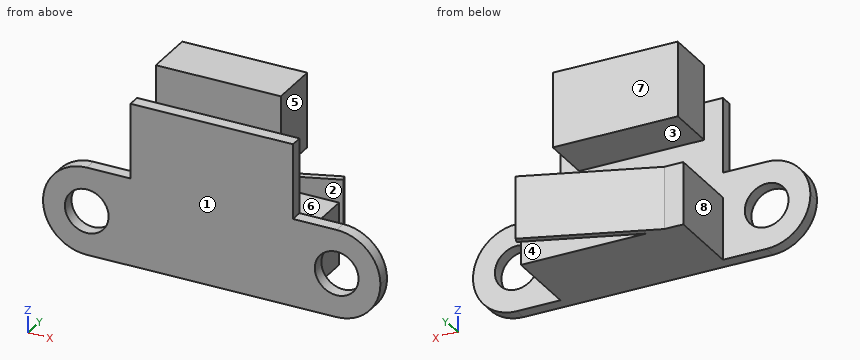
from build123d import *

# Parameters (mm, degrees)
SKETCH1_W           = 13
SKETCH1_H           = 13
BOSS_EXTRUDE1_DEPTH = 1
SKETCH4_W           = 7
SKETCH4_H           = 1
BOSS_EXTRUDE2_DEPTH = 7
SKETCH5_W           = 7
SKETCH5_H           = 1
BOSS_EXTRUDE3_DEPTH = 7
SKETCH6_R           = 1.75
CUT_EXTRUDE1_DEPTH  = 16.016657418
SKETCH7_W           = 10
SKETCH7_H           = 6
BOSS_EXTRUDE4_DEPTH = 4
SKETCH8_W           = 13
SKETCH8_H           = 5
BOSS_EXTRUDE5_DEPTH = 6
BOSS_EXTRUDE6_DEPTH = 5
FILLET1_R           = 3.5


with BuildPart() as part:
    # Sketch1 → Boss-Extrude1 (new body)
    with BuildSketch(Plane(origin=(0, 0, 0), x_dir=(1, 0, 0), z_dir=(0, 1, 0))):
        Rectangle(SKETCH1_W, SKETCH1_H)
    extrude(amount=BOSS_EXTRUDE1_DEPTH)

    # Sketch4 → Boss-Extrude2 (add)
    with BuildSketch(Plane.ZY.offset(6.5)):
        with Locations((-3, 0.5)):
            Rectangle(SKETCH4_W, SKETCH4_H)
    extrude(amount=BOSS_EXTRUDE2_DEPTH)

    # Sketch5 → Boss-Extrude3 (add)
    with BuildSketch(Plane(origin=(6.5, 0, 0), x_dir=(0, 0, -1), z_dir=(1, 0, 0))):
        with Locations((3, 0.5)):
            Rectangle(SKETCH5_W, SKETCH5_H)
    extrude(amount=BOSS_EXTRUDE3_DEPTH)

    # Sketch6 → Cut-Extrude1 (cut, through all)
    with BuildSketch(Plane(origin=(0, 1, 0), x_dir=(1, 0, 0), z_dir=(0, 1, 0))):
        with Locations(Location((-10, 3, 0), (0, 0, 270))):
            Circle(SKETCH6_R)
        with Locations(Location((10, 3, 0), (0, 0, 270))):
            Circle(SKETCH6_R)
    extrude(amount=-CUT_EXTRUDE1_DEPTH, mode=Mode.SUBTRACT)

    # Sketch7 → Boss-Extrude4 (add)
    with BuildSketch(Plane(origin=(0, 1, 0), x_dir=(1, 0, 0), z_dir=(0, 1, 0))):
        with Locations((0, -6.5)):
            Rectangle(SKETCH7_W, SKETCH7_H)
    extrude(amount=BOSS_EXTRUDE4_DEPTH)

    # Sketch8 → Boss-Extrude5 (add)
    with BuildSketch(Plane(origin=(0, 1, 0), x_dir=(1, 0, 0), z_dir=(0, 1, 0))):
        with Locations((0, 4)):
            Rectangle(SKETCH8_W, SKETCH8_H)
    extrude(amount=BOSS_EXTRUDE5_DEPTH)

    # Sketch9 → Boss-Extrude6 (add)
    with BuildSketch(Plane.XY.offset(-1.5)):
        Polygon((-5, 7), (5, 10.639702343), (5.171010072, 10.169856032), (-3.5380978, 7), align=None)
    extrude(amount=-BOSS_EXTRUDE6_DEPTH)

    # Fillet1
    fillet1_edges = [part.edges().sort_by_distance(p)[0] for p in [
        (13.5, 0.5, -6.5),
        (13.5, 0.5, 0.5),
        (-13.5, 0.5, -6.5),
        (-13.5, 0.5, 0.5),
    ]]
    fillet(fillet1_edges, radius=FILLET1_R - 0.0001)  # a hair under: the kernel refuses the full size


solid = part.part
Can you work these out from the model? Positions are in its coordinate system, mm. Face numbers are marked on the shaded views. A direction names the side the tool comes from. Give positions to 0.01 mm unless a question says otherwise; leave off trailing zeros. Order: outer loops, then holes, each group sorted by start corner. A loop starts at its lowest first (then second) coordinate and runs counter-clockwise, first axis right, second up. Notation, with made-up numbers: (86, 6.25) - (108, 6.25) arc R21 ccw to (108, 24.25) - close; hole circle Ø8 at (14, 15.5). An arc over 180 degrees is marked (long way). Write each question's results on one line, items separated by ' | '.
1) If we mould it in two halves opening along Y, with no side actions, what happens to the marked faces 1, 2, 3 and 4? For each: pulls with the +Y half, pulls with the -Y half, needs draft (parallel to the pull), parting line crosses it, or undercut.
Final values:
face 1: pulls with the -Y half | face 2: undercut | face 3: needs draft | face 4: undercut
2) I'm going to push flat-ended pins straight in: pin 1 Ø3 at (x, y) = (6, 1) entering from +Z; pin 2 Ø1.8 at (x, z) = (0, 6) entering from +Y; pin 3 Ø1.5 at (x, z) = (1, 7.5) entering from -Y; pin 4 Ø4 at (y, z) = (7, 3) entering from -X. Where does each tip first touch, or does it pass through?
Final values:
pin 1: stops at z = 9.5 | pin 2: stops at y = 5 | pin 3: stops at y = 1 | pin 4: passes through
3) Suppose I cut it at B-B, the plane z = -4. Write out the boundary of the cut face in (x, y).
Final values:
outline: (-13.35, 0) - (-11.44, 0) - (-11.44, 1) - (-13.35, 1) - close; (-8.56, 0) - (8.56, 0) - (8.56, 1) - (6.5, 1) - (6.5, 7) - (-3.54, 7) - (5.17, 10.17) - (5, 10.64) - (-5, 7) - (-6.5, 7) - (-6.5, 1) - (-8.56, 1) - close; (11.44, 0) - (13.35, 0) - (13.35, 1) - (11.44, 1) - close
4) Suppose I cut it at C-C, the plane y = 5.75. Write out the boundary of the cut face in (x, z), then the cut area to 3 significant figures.
Final values:
outline: (-6.5, -6.5) - (6.5, -6.5) - (6.5, -1.5) - (-6.5, -1.5) - close | area: 65.0 mm^2
5) Suppose I cut it at D-D, the plane x = 10.5. Write out the boundary of the cut face in (y, z).
Final values:
outline: (0, -6.46) - (1, -6.46) - (1, -4.68) - (0, -4.68) - close; (0, -1.32) - (1, -1.32) - (1, 0.46) - (0, 0.46) - close
6) Please list where these lines run through material, in increasing order: line 1 along X through (y, z) = (0.75, -3); line 2 along X through (y, z) = (3, 8); line 3 along Y through (x, z) = (4.5, 2.75). Write a range as [from, to].
Final values:
line 1: x = [-13.5, -11.75], [-8.25, 8.25], [11.75, 13.5] | line 2: x = [-5, 5] | line 3: y = [0, 1]
7) Suppose I cut it at A-A, the plane x = 4.25. Write out the boundary of the cut face in (y, z), then the cut area to 3 significant figures.
Final values:
outline: (0, -6.5) - (7, -6.5) - (7, -1.5) - (1, -1.5) - (1, 3.5) - (5, 3.5) - (5, 9.5) - (1, 9.5) - (1, 6.5) - (0, 6.5) - close; (9.83, -6.5) - (10.37, -6.5) - (10.37, -1.5) - (9.83, -1.5) - close | area: 69.7 mm^2
8) On a 3-axis mill with a long thin cutter (end or side, diameter ignored), from which of +Z, -Z, +X, -X, +Y, -Y can I reach the whole of each face in a straight line? I mean the marked faces 5, 6, 7 and 8. Say none if no direction works.
Final values:
face 5: +Z, +X, +Y | face 6: +X, -X, +Y | face 7: +Z, +X, -X, +Y | face 8: +Z, -Z, -X, +Y
